Design review of the part built by this model. Coordinates are the model's own, in mm. A direction names the side the tool comes from. Round coordinates to 2 decimals unless told otherwise and drop trailing zeros. Loops run counter-clockwise (first coordinate to the right, second up) from the corner with the lowest first, then second, coordinate; pieces in that order, holes last. Notation, with made-up numbers: M 10.5,77 L 66.5,77 A10 cw 66.5,91 Z; hole C -11,53.5 d4. An arc over 180 degrees is marked long. One line per item, written item: value. Start each with the question number.
Item 1: For line 1 along Y through (x, z) = (0, -5.1); line 2 along Z through (x, y) = (-1.75, -2), list the stretches that pass through material, from the lowest coordinate up.
Item 2: We need section A-A (x = 0). State how many separate pieces and enclosed holes the cut face has, then the cut area to 3 significant figures.
Item 3: For faces 1 (the cylindrical face through (-0.215, 14.337, -4.418)), 2 (the flat face through (2.9, 10.7, 0)), 3 (the flat face through (0, 16.002, -1)), 4 (the cylindrical face through (0.762, -4.418, 14.165)), 5 (the flat face through (0, -2.54, 9)), list the 3-axis set-ups (+Z, -Z, +X, -X, +Y, -Y) from which the entire face can be reached by the end or side of a thin tool; tool diameter is ignored.
Item 4: Clearance check with flat-ended pins moving along their axes: pin 1 (6 mm diameter, centred on x = 0.5, y = 7.5, fed in from +Z); pin 2 (2.5 mm diameter, centred on x = 0, z = 6.5, fed in from +Y); pin 3 (3 mm diameter, centred on x = -5, z = 7, fed in from +Y). State where each tip first meets the part, or that it passes through.
Item 5: We need section C-C (z = 5.5). Write out the cut boundary in (x, y).
Item 6: We need section B-B (y = -4.5). Write out the cut boundary in (x, z), then the cut area to 3 significant figures.
Item 7: Mouldability with a two-part tool opening along Y and no side actions: class faces 6 (the flat face through (0, -6.35, 3)), 7 (the flat face through (2.909, -1.252, 11.135)), 8 (the cylindrical face through (0, 8, -4)) as released by +Y, released by -Y, zero draft, split by the parting line, or undercut.
Item 8: We need section D-D (y = 14). Write out the cut boundary in (x, z).
from build123d import *

# Parameters (mm, degrees)
BOSS_EXTRUDE1_DEPTH      = 6.35
BOSS_EXTRUDE1_DEPTH_BACK = 6.35
SKETCH2_R                = 1.651
CUT_EXTRUDE1_DEPTH       = 25.4
CUT_EXTRUDE2_DEPTH       = 2.54
SKETCH4_R                = 1.651
CUT_EXTRUDE3_DEPTH       = 6.35
CUT_EXTRUDE4_DEPTH       = 2.54
CHAMFER1_SIZE            = 2.54
FILLET1_R                = 2.54


with BuildPart() as part:
    # Sketch1 → Boss-Extrude1 (new body, two sides)
    with BuildSketch(Plane(origin=(0, 0, 0), x_dir=(0, 0, -1), z_dir=(1, 0, 0))) as boss_extrude1_sk:
        Polygon((0, 0), (0, 19.05), (6.35, 19.05), (6.35, -6.35), (-19.05, -6.35), (-19.05, 0), align=None)
    extrude(amount=BOSS_EXTRUDE1_DEPTH)
    extrude(boss_extrude1_sk.sketch, amount=-BOSS_EXTRUDE1_DEPTH_BACK)

    # Sketch2 → Cut-Extrude1 (cut)
    with BuildSketch(Plane(origin=(0, 0, 0), x_dir=(1, 0, 0), z_dir=(0, 1, 0))):
        with Locations((0, -6.35)):
            Circle(SKETCH2_R)
        with Locations((0, -12.7)):
            Circle(SKETCH2_R)
    extrude(amount=-CUT_EXTRUDE1_DEPTH, mode=Mode.SUBTRACT)

    # Sketch3 → Cut-Extrude2 (cut)
    with BuildSketch(Plane(origin=(0, 0, 0), x_dir=(1, 0, 0), z_dir=(0, 1, 0))):
        Polygon((1.906410589, -3.048), (-1.906410589, -3.048), (-3.812821178, -6.35), (-1.979734073, -9.525), (-3.812821178, -12.7), (-1.906410589, -16.002), (1.906410589, -16.002), (3.812821178, -12.7), (1.979734073, -9.525), (3.812821178, -6.35), align=None)
    extrude(amount=-CUT_EXTRUDE2_DEPTH, mode=Mode.SUBTRACT)

    # Sketch4 → Cut-Extrude3 (cut)
    with BuildSketch(Plane.XY):
        with Locations((0, 12.7)):
            Circle(SKETCH4_R)
        with Locations((0, 6.35)):
            Circle(SKETCH4_R)
    extrude(amount=-CUT_EXTRUDE3_DEPTH, mode=Mode.SUBTRACT)

    # Sketch5 → Cut-Extrude4 (cut)
    with BuildSketch(Plane.XY):
        Polygon((1.906410589, 16.002), (-1.906410589, 16.002), (-3.812821178, 12.7), (-1.979734073, 9.525), (-3.812821178, 6.35), (-1.906410589, 3.048), (1.906410589, 3.048), (3.812821178, 6.35), (1.979734073, 9.525), (3.812821178, 12.7), align=None)
    extrude(amount=-CUT_EXTRUDE4_DEPTH, mode=Mode.SUBTRACT)

    # Chamfer1
    chamfer1_edges = [part.edges().sort_by_distance(p)[0] for p in [
        (0, 0, 0),
    ]]
    chamfer(chamfer1_edges, length=CHAMFER1_SIZE)

    # Fillet1
    fillet1_edges = [part.edges().sort_by_distance(p)[0] for p in [
        (6.35, -3.175, 19.05),
        (6.35, 19.05, -3.175),
        (-6.35, 19.05, -3.175),
        (-6.35, -3.175, 19.05),
    ]]
    fillet(fillet1_edges, radius=FILLET1_R)


solid = part.part
A:
1. line 1: -6.35 to 4.7, 8 to 11.05, 14.35 to 19.05
1. line 2: -6.35 to 3.05, 16 to 19.05
2. separate pieces: 5
2. enclosed holes: 0
2. area: 169 mm2
3. face 1: +Z, -Z
3. face 2: +Z, +X, -X, +Y
3. face 3: +Z
3. face 4: +Y, -Y
3. face 5: +Y
4. pin 1: z = 0
4. pin 2: through
4. pin 3: y = 0
5. outline: M -6.35,-6.35 L -1.42,-6.35 L -1.42,-2.54 L -3.32,-2.54 L -3.32,0 L -6.35,0 Z; M 1.42,-6.35 L 6.35,-6.35 L 6.35,0 L 3.32,0 L 3.32,-2.54 L 1.42,-2.54 Z
6. outline: M -6.35,-6.35 L 6.35,-6.35 L 6.35,16.51 A2.54 ccw 3.81,19.05 L -3.81,19.05 A2.54 ccw -6.35,16.51 Z; hole C 0,6.35 d3.3; hole C 0,12.7 d3.3
6. area: 303 mm2
7. face 6: released by -Y
7. face 7: zero draft
7. face 8: undercut
8. outline: M -6.35,-6.35 L -1.02,-6.35 L -1.02,-2.54 L -3.06,-2.54 L -3.06,0 L -6.35,0 Z; M 1.02,-6.35 L 6.35,-6.35 L 6.35,0 L 3.06,0 L 3.06,-2.54 L 1.02,-2.54 Z
